```python
from build123d import *

# Parameters (mm, degrees)
F0_W     = 480
F0_H     = 480
F1_DEPTH = 90
F0_W_2   = 65.4
F0_H_2   = 100
F0_W_3   = 130.8
F2_DEPTH = 90


with BuildPart() as f1:
    # F0 (on Front) → F1 (new body)
    with BuildSketch(Plane.XZ):
        Rectangle(F0_W, F0_H)
        Polygon((-170.8, -236.2), (-236.2, -236.2), (-236.2, -136.2), (-236.2, 236.2), (236.2, 236.2), (236.2, -136.2), (236.2, -236.2), (105.4, -236.2), align=None, mode=Mode.SUBTRACT)
    extrude(amount=F1_DEPTH)

    # F0 (on Front) → F2 (join)
    with BuildSketch(Plane.XZ):
        with Locations((-203.5, -186.2)):
            Rectangle(F0_W_2, F0_H_2)
        with Locations((170.8, -186.2)):
            Rectangle(F0_W_3, F0_H_2)
    extrude(amount=F2_DEPTH)


solid = f1.part
```
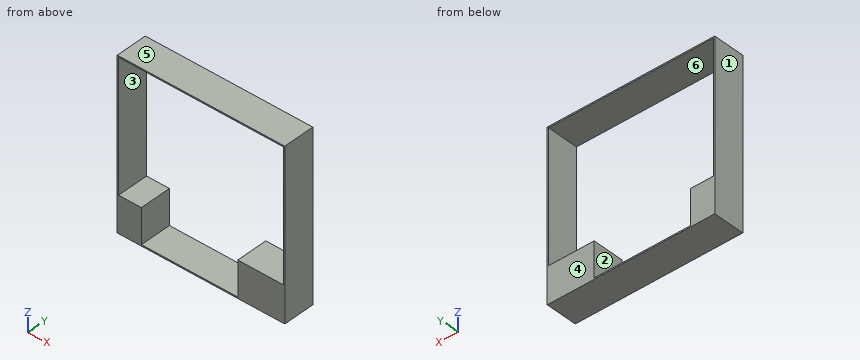
Can you work these out from the model? Positions are in its coordinate system, mm. Face numbers are marked on the shaded views. A direction names the side the tool comes from. Coordinates: 2 decimals unless noted, no trailing zeros. Loops run counter-clockwise (first coordinate to the right, second up) from the corner with the lowest first, then second, coordinate; pieces in that order, holes last. Notation, with made-up numbers: (40.5, 84.5) - (90.5, 84.5) arc R8 ccw to (90.5, 90.5) - close; hole circle Ø3 at (51.5, 48.5). An arc over 180 degrees is marked (long way). Use a Markdown table: item, result.
Item 1: I want a section at C-C on y = -62. Please give me the cut outline in (x, z), and give its area (3 significant figures).
Numbers:
| item | result |
|---|---|
| outline | (-240, -240) - (240, -240) - (240, 240) - (-240, 240) - close; hole (-236.2, -136.2) - (-170.8, -136.2) - (-170.8, -236.2) - (105.4, -236.2) - (105.4, -136.2) - (236.2, -136.2) - (236.2, 236.2) - (-236.2, 236.2) - close |
| area | 26,900 mm2 |
Item 2: If I drill on probe 1 along X at (y, z) = (-30, -134); probe 2 along Z at (x, y) = (-171.5, -71), over which ranges is the centre line in solid material (lowest first)? Write a range as from..to.
Numbers:
| item | result |
|---|---|
| probe 1 | x = -240..-236.2, 236.2..240 |
| probe 2 | z = -240..-136.2, 236.2..240 |
Item 3: I want a section at B-B on x = 33. Please give me the cut outline in (y, z).
Numbers:
| item | result |
|---|---|
| outline | (-90, -240) - (0, -240) - (0, -236.2) - (-90, -236.2) - close; (-90, 236.2) - (0, 236.2) - (0, 240) - (-90, 240) - close |
Item 4: For the marked faces 1 and 2, which set-ups out of +Z, -Z, +X, -X, +Y, -Y let a thin tool reach every point of the face, with its end or its side?
Numbers:
| item | result |
|---|---|
| face 1 | +Z, -Z, -X, +Y, -Y |
| face 2 | +Y, -Y |
Item 5: I want a section at A-A on z = 176.5. Please give me the cut outline in (x, y).
Numbers:
| item | result |
|---|---|
| outline | (-240, -90) - (-236.2, -90) - (-236.2, 0) - (-240, 0) - close; (236.2, -90) - (240, -90) - (240, 0) - (236.2, 0) - close |
Item 6: We'd pull the mould along Z, two halves only. Please class the marked faces 3, 4, 5 and 6: released by +Z, released by -Z, zero draft, split by the parting line, or undercut.
Numbers:
| item | result |
|---|---|
| face 3 | undercut |
| face 4 | zero draft |
| face 5 | released by +Z |
| face 6 | undercut |
